For this review, take the finished solid that the model builds, in its own axes (mm). A direction names the side the tool comes from. Give positions to 0.01 mm unless a question says otherwise; leave off trailing zeros. Loops run counter-clockwise (first coordinate to the right, second up) from the corner with the lowest first, then second, coordinate; pieces in that order, holes last.
```python
from build123d import *

# Parameters (mm, degrees)
SKETCH1_R            = 18.5039
GEARBOX_DEPTH        = 26.0096
SKETCH2_R            = 17.8943
BOSS_EXTRUDE2_DEPTH  = 56.9976
SKETCH3_R            = 18.9992
WRAP_DEPTH           = 33.6804
SKETCH4_R            = 18.4277
BOSS_EXTRUDE4_DEPTH  = 24.501601563
CONNECTDOR_START     = -6.5786
CONNECTDOR_CUT_DEPTH = 6.5786
SKETCH6_R            = 11.9888
CENTER_DISH_DEPTH    = 0.635
SKETCH7_R            = 7.62
BOSS_EXTRUDE5_DEPTH  = 0.635
CHAMFER4_SIZE        = 0.635
CHAMFER5_SIZE        = 0.635
SKETCH8_R            = 6.05155
SHAFT_COLLAR_DEPTH   = 6.7056
FILLET1_R            = 0.396875
SKETCH9_R            = 2.9972
BOSS_EXTRUDE7_DEPTH  = 25.8318
CUT_EXTRUDE3_START   = -22.225
CUT_EXTRUDE3_DEPTH   = 22.225


with BuildPart() as part:
    # Sketch1 → Gearbox (new body)
    with BuildSketch(Plane.XY):
        Circle(SKETCH1_R)
    extrude(amount=-GEARBOX_DEPTH)

    # Sketch2 → Boss-Extrude2 (add)
    with BuildSketch(Plane(origin=(0, 0, -26.0096), x_dir=(-1, 0, 0), z_dir=(0, 0, -1))):
        with Locations(Location((0, 0, 0), (0, 0, 180))):
            Circle(SKETCH2_R)
    extrude(amount=BOSS_EXTRUDE2_DEPTH)

    # Sketch3 → Wrap (add)
    with BuildSketch(Plane(origin=(0, 0, -29.9974), x_dir=(-1, 0, 0), z_dir=(0, 0, -1))):
        Circle(SKETCH3_R)
    extrude(amount=WRAP_DEPTH)

    # Sketch4 → Boss-Extrude4 (add)
    with BuildSketch(Plane(origin=(0, 0, -83.0072), x_dir=(-1, 0, 0), z_dir=(0, 0, -1))):
        with Locations(Location((0, 0, 0), (0, 0, 180))):
            Circle(SKETCH4_R)
    extrude(amount=BOSS_EXTRUDE4_DEPTH)

    # Connector → Connectdor Cut (cut)
    with BuildSketch(Plane(origin=(0, 0, -107.508801563), x_dir=(-1, 0, 0), z_dir=(0, 0, -1)).offset(CONNECTDOR_START)):
        with BuildLine():
            Line((0, 8.001), (16.600124285, 8.001))
            ThreePointArc((16.600124285, 8.001), (0, 18.4277), (-16.600124285, 8.001))
            Line((-16.600124285, 8.001), (0, 8.001))
        make_face()
    extrude(amount=CONNECTDOR_CUT_DEPTH, mode=Mode.SUBTRACT)

    # Sketch6 → Center DIsh (cut)
    with BuildSketch(Plane.XY):
        Circle(SKETCH6_R)
    extrude(amount=-CENTER_DISH_DEPTH, mode=Mode.SUBTRACT)

    # Sketch7 → Boss-Extrude5 (add)
    with BuildSketch(Plane.XY.offset(-0.635)):
        with Locations((0, 7.0104)):
            Circle(SKETCH7_R)
    extrude(amount=BOSS_EXTRUDE5_DEPTH)

    # Chamfer4
    chamfer4_edges = [part.edges().sort_by_distance(p)[0] for p in [
        (0, -0.6096, -0.635),
    ]]
    chamfer(chamfer4_edges, length=CHAMFER4_SIZE - 0.0001)  # a hair under: the kernel refuses the full size

    # Chamfer5
    chamfer5_edges = [part.edges().sort_by_distance(p)[0] for p in [
        (0, -11.9888, -0.635),
    ]]
    chamfer(chamfer5_edges, length=CHAMFER5_SIZE - 0.0001)  # a hair under: the kernel refuses the full size

    # Sketch8 → Shaft Collar (add)
    with BuildSketch(Plane.XY):
        with Locations((0, 7.92156223)):
            Circle(SKETCH8_R)
    extrude(amount=SHAFT_COLLAR_DEPTH)

    # Fillet1
    fillet1_edges = [part.edges().sort_by_distance(p)[0] for p in [
        (-6.05155, 7.92156223, 6.7056),
    ]]
    fillet(fillet1_edges, radius=FILLET1_R)

    # Sketch9 → Boss-Extrude7 (add)
    with BuildSketch(Plane.XY.offset(6.7056)):
        with Locations((0, 7.92156223)):
            Circle(SKETCH9_R)
    extrude(amount=BOSS_EXTRUDE7_DEPTH)

    # Sketch10 → Cut-Extrude3 (cut)
    with BuildSketch(Plane.XY.offset(32.5374).offset(CUT_EXTRUDE3_START)):
        with BuildLine():
            Line((0, 10.35996223), (-1.742817627, 10.35996223))
            ThreePointArc((-1.742817627, 10.35996223), (0, 10.91876223), (1.742817627, 10.35996223))
            Line((1.742817627, 10.35996223), (0, 10.35996223))
        make_face()
    extrude(amount=CUT_EXTRUDE3_DEPTH, mode=Mode.SUBTRACT)


solid = part.part
```
Q1. For pin 1 Ø1.5 at (y, z) = (-15, -86.5) entering from -X; pin 2 Ø8 at (y, z) = (-1, -2) entering from +X; pin 3 Ø5 at (y, z) = (15, -67.5) entering from -X; pin 4 Ø12 at (x, z) = (-14.5, 13.5) entering from +Y, all flat-tipped, find the tip position at first contact; note any pin that passes through.
Answers:
pin 1: stops at x = -11.68
pin 2: stops at x = 18.5
pin 3: stops at x = -12.8
pin 4: passes through
Q2. Machinability: for faces 1 (the flat face through (2, 5, 6.706)), 2 (the flat face through (0, 10.36, 21)), 3 (the flat face through (13, -13, -63.678)), which of the approach directions +Z, -Z, +X, -X, +Y, -Y give a long, thin tool a straight path to every point of the face, cutting with its end or side? Answer none if there is none.
Answers:
face 1: +Z
face 2: +Z, +X, -X, +Y
face 3: none
Q3. Consider section C-C on z = -98.5. Give the boundary of the cut face in (x, y), plus the area to 3 significant figures.
Answers:
outline: circle Ø36.86 at (0, 0)
area: 1,070 mm2
Q4. Mouldability with a two-part tool opening along X and no side actions: class faces 4 (the flat face through (-3, -18, -83.007)), 5 (the cylindrical face through (-4.011, -18.064, -12.823)), 6 (the flat face through (0, -4, -0.635)) as +X half, -X half, draft (parallel to the pull), parting line (faces both ways), or undercut.
Answers:
face 4: draft
face 5: parting line
face 6: undercut
Q5. Consider section B-B on y = -15.5. Give the boundary of the cut face in (x, z), plus the area to 3 significant figures.
Answers:
outline: (-10.99, -63.68) - (-8.94, -63.68) - (-8.94, -83.01) - (-9.97, -83.01) - (-9.97, -107.51) - (9.97, -107.51) - (9.97, -83.01) - (8.94, -83.01) - (8.94, -63.68) - (10.99, -63.68) - (10.99, -30) - (8.94, -30) - (8.94, -26.01) - (10.11, -26.01) - (10.11, 0) - (-10.11, 0) - (-10.11, -26.01) - (-8.94, -26.01) - (-8.94, -30) - (-10.99, -30) - close
area: 2,170 mm2
Q6. Consider section A-A on z = -19. Give the boundary of the cut face in (x, y), plus the area to 3 significant figures.
Answers:
outline: circle Ø37.01 at (0, 0)
area: 1,080 mm2
Q7. For probe 1 along Z at (x, y) = (-9, -16); probe 2 along Z at (x, y) = (2.5, -15); probe 3 along Z at (x, y) = (0.5, 2.5), list the stretches that pass through material, from the lowest coordinate up.
Answers:
probe 1: z = -107.51 to -83.01, -63.68 to -30, -26.01 to 0
probe 2: z = -107.51 to 0
probe 3: z = -107.51 to 6.71
